from build123d import *

# Parameters (mm, degrees)
F3_W        = 23.168018
F3_H        = 27.206479
F3_W_2      = 23.380567
F3_H_2      = 21.892714
F4_DEPTH    = 4
F1_FACE_R   = 30.911156
F1_FACE_R_2 = 27.45
F5_DEPTH    = 1.5


with BuildPart() as f1:
    # F0 (on Front) → F1 (revolve)
    with BuildSketch(Plane.XZ):
        with BuildLine():
            Line((-28.734368, 1.925376), (-30.911156, 0))
            Line((-30.911156, 0), (-27.45, 0))
            ThreePointArc((-27.45, 0), (-27.273223, 0.073223), (-27.2, 0.25))
            Line((-27.2, 0.25), (-27.2, 5))
            Line((-27.2, 5), (-27.2, 9.999887))
            Line((-27.2, 9.999887), (-27.2, 11.112636))
            Line((-27.2, 11.112636), (-28.65, 11.112636))
            Line((-28.65, 11.112636), (-28.65, 2.112636))
            ThreePointArc((-28.65, 2.112636), (-28.672066, 2.009942), (-28.734368, 1.925376))
        make_face()
    revolve(axis=Axis((0, 0, 10.43564), (0, 0, -1)))

    # F3 (on offset) → F4 (cut)
    with BuildSketch(Plane.XY.offset(8.8)):
        with Locations((0, 24.549596)):
            Rectangle(F3_W, F3_H)
        with Locations((-23.274293, 0)):
            Rectangle(F3_W_2, F3_H_2)
        with Locations((23.274293, 0)):
            Rectangle(F3_W_2, F3_H_2)
        with Locations((0, -24.549596)):
            Rectangle(F3_W, F3_H)
    extrude(amount=F4_DEPTH, mode=Mode.SUBTRACT)

    # F1_face (on face) → F5 (join)
    with BuildSketch(Plane(origin=(0, 0, 0), x_dir=(1, 0, 0), z_dir=(0, 0, -1))):
        Circle(F1_FACE_R)
        Circle(F1_FACE_R_2, mode=Mode.SUBTRACT)
    extrude(amount=F5_DEPTH)


solid = f1.part
Design review of the part built by this model. Coordinates are the model's own, in mm. A direction names the side the tool comes from. Coordinates: 2 decimals unless noted, no trailing zeros. Loops run counter-clockwise (first coordinate to the right, second up) from the corner with the lowest first, then second, coordinate; pieces in that order, holes last. Notation, with made-up numbers: M 9.25,80 L 56.25,80 A28 cw 56.25,118 Z; hole C 56.5,37 d6. An arc over 180 degrees is marked long. Answer as CSV lines item,"result".
Item 1: Add section C-C on z = 1. State the section outline as (x, y) points, plus the area to 3 significant figures.
Answer list:
outline,"C 0,0 d59.56; hole C 0,0 d54.4"
area,"462 mm²"
Item 2: For P1, Ø3, axis at x = -27, y = -0.5, coming from the +Z side; P2, Ø1.3, axis at y = 25, z = 10.5, coming from the +X side; P3, Ø2, axis at x = -6.5, z = 2, coming from the +Y side; P4, Ø10, axis at x = -14, y = 12.5, coming from the -Z side, all flat-tipped, find the tip position at first contact; note any pin that passes through.
Answer list:
P1,"z = 8.8"
P2,"x = 15.1"
P3,"y = 29.08"
P4,"through"
Item 3: For probe 1 along Y at (x, z) = (0, -0.5); probe 2 along Y at (x, z) = (0, 7), list the stretches that pass through material, from the lowest coordinate up.
Answer list:
probe 1,"-30.91 to -27.45, 27.45 to 30.91"
probe 2,"-28.65 to -27.2, 27.2 to 28.65"
Item 4: Add section A-A on x = 0. State the section outline as (y, z) points, plus the area to 3 significant figures.
Answer list:
outline,"M -30.91,-1.5 L -27.45,-1.5 L -27.45,0 A0.25 ccw -27.2,0.25 L -27.2,8.8 L -28.65,8.8 L -28.65,2.11 A0.25 cw -28.73,1.93 L -30.91,0 Z; M 27.2,0.25 A0.25 ccw 27.45,0 L 27.45,-1.5 L 30.91,-1.5 L 30.91,0 L 28.73,1.93 A0.25 cw 28.65,2.11 L 28.65,8.8 L 27.2,8.8 Z"
area,"40.4 mm²"
Item 5: Machinability: for faces 4 (the face through (20, 19, 11.113)), 5 (the face through (26, -10.946, 10)), 6 (the face through (26.18, -8.25, -0.74)), 7 (the face through (11.584, -25, 10)), 8 (the face through (6.259, -28.184, 1.805)), which of the approach directions +Z, -Z, +X, -X, +Y, -Y give a long, thin tool a straight path to every point of the face, cutting with its end or side? Answer none if there is none.
Answer list:
face 4,"+Z, +X, -X, +Y, -Y"
face 5,"+Z, +X, -X"
face 6,"-Z"
face 7,"+Z, +Y, -Y"
face 8,"+Z"
Item 6: The part is to be moulded in two halves that separate along X. For faces 1 (the face through (28.554, 11.839, -0.74)), 2 (the face through (11.584, 25, 10)), 3 (the face through (0, -28, -1.5)), say which applies: pulls with the +X half, pulls with the -X half, needs draft (parallel to the pull), parting line crosses it, or undercut.
Answer list:
face 1,"parting line crosses it"
face 2,"undercut"
face 3,"needs draft"
